Could you check a few things on this model? Use its own coordinates, in mm. Give positions to 0.01 mm unless a question says otherwise; leave off trailing zeros. Loops run counter-clockwise (first coordinate to the right, second up) from the corner with the lowest first, then second, coordinate; pieces in that order, holes last. Notation, with made-up numbers: (11, -19.5) - (44, -19.5) arc R31 ccw to (44, 9.5) - close; hole circle Ø2 at (35.5, -2). An arc over 180 degrees is marked (long way). Write each question's results on one line, items separated by ' | '. Start each with the question number.
1) If we mould it in two halves opening along Y, with no side actions, what happens to faces 1 (the face through (-130.505, 0.242, -2.412)), 2 (the face through (-3, 6, -5))? For each: +Y half, -Y half, draft (parallel to the pull), parting line (faces both ways), or undercut.
2) I'm going to push flat-ended pins straight in: pin 1 (1 mm diameter, centred on y = -10.5, z = -3.5, fed in from +X); pin 2 (7 mm diameter, centred on x = 0, y = 0, fed in from +Z). Where does each tip first touch, or does it pass through?
3) If I drill on probe 1 along Y at (x, z) = (60, -2.4); probe 2 along Y at (x, z) = (0, 3); probe 3 along Z at (x, y) = (-53, 3.5), over which ranges is the centre line in solid material (lowest first)? Write a range as [from, to].
4) I want a section at A-A, the plane x = -136. Write out the boundary of the cut face in (y, z).
from build123d import *

# Parameters (mm, degrees)
F0_W           = 380
F0_H           = 52.2
F1_DEPTH       = 5
F2_SIZE        = 2.5
F4_D           = 6
F5_D           = 11
F5_CSINK_D     = 20.5
F5_CSINK_ANGLE = 90


with BuildPart() as f1:
    # F0 (on Top) → F1 (new body, symmetric)
    with BuildSketch(Plane.XY):
        Rectangle(F0_W, F0_H)
    extrude(amount=F1_DEPTH, both=True)

    # F2
    f2_edges = [f1.edges().sort_by_distance(p)[0] for p in [
        (0, 26.1, 5),
        (-190, 0, 5),
        (0, -26.1, 5),
        (190, 0, 5),
        (0, 26.1, -5),
        (-190, 0, -5),
        (0, -26.1, -5),
        (190, 0, -5),
    ]]
    chamfer(f2_edges, length=F2_SIZE)

    # F4 (through all)
    with Locations(Plane.XY.offset(5)):
        with Locations((0, 0)):
            Hole(F4_D / 2)

    # F5 (through all)
    with Locations(Plane.XY.offset(5)):
        with Locations((-136, 0), (-60, 0), (60, 0), (136, 0)):
            CounterSinkHole(F5_D / 2, F5_CSINK_D / 2, counter_sink_angle=F5_CSINK_ANGLE)


solid = f1.part
Answers:
1) face 1: undercut | face 2: draft
2) pin 1: stops at x = 189.5 | pin 2: stops at z = 5
3) probe 1: y = [-26.1, -5.5], [5.5, 26.1] | probe 2: y = [-25.6, -3], [3, 25.6] | probe 3: z = [-5, 2.58]
4) outline: (-26.1, -2.5) - (-23.6, -5) - (-5.5, -5) - (-5.5, 0.25) - (-10.25, 5) - (-23.6, 5) - (-26.1, 2.5) - close; (5.5, -5) - (23.6, -5) - (26.1, -2.5) - (26.1, 2.5) - (23.6, 5) - (10.25, 5) - (5.5, 0.25) - close
